Model file for the job. Use its own axes, mm. A direction names the side the tool comes from. Round coordinates to 2 decimals unless told otherwise and drop trailing zeros. Loops run counter-clockwise (first coordinate to the right, second up) from the corner with the lowest first, then second, coordinate; pieces in that order, holes last.
Autodesk Inventor part; units mm, degrees
ref_plane "YZ Plane" through (0, 0, 0) normal (1, 0, 0) x (0, 1, 0)
ref_plane "XZ Plane" through (0, 0, 0) normal (0, 1, 0) x (-1, 0, 0)
ref_plane "XY Plane" through (0, 0, 0) normal (0, 0, 1) x (1, 0, 0)
sketch "Sketch1" plane through (0, 0, 0) normal (0, 1, 0) x (-1, 0, 0)
  circle A0 centre (0, 0) radius 14.986
  dimension "d0" = 29.972
extrude "Extrusion1" add sketch "Sketch1" along normal mid plane 99.06
sketch "Sketch2" plane through (0, 0, 0) normal (1, 0, 0) x (0, 1, 0)
  line L0 (-49.53, 14.986) -> (-49.53, -14.986)
  line L1 (49.53, -14.986) -> (49.53, 14.986)
  line L2 (0, 14.986) -> (0, -71.9195) construction
  line L3 (49.53, 14.986) -> (49.53, -46.736)
  line L4 (49.53, -46.736) -> (111.252, -46.736)
  line L5 (111.252, -46.736) -> (49.53, 14.986)
  line L6 (-49.53, -14.986) -> (-49.53, 14.986)
  line L7 (-49.53, 14.986) -> (-49.53, -46.736)
  line L8 (-49.53, -46.736) -> (-111.252, -46.736)
  line L9 (-111.252, -46.736) -> (-49.53, 14.986)
  point P0 (0, 0)
  dimension "d3" = 61.722
  dimension "d4" = 61.722
extrude "Extrusion2" add sketch "Sketch2" along normal mid plane 25.4
sketch "Sketch3" plane through (12.7, 111.252, -46.736) normal (0, 0, -1) x (-1, 0, 0)
  line L0 (12.7, -111.252) -> (12.7, -6.477) construction
  circle A0 centre (12.7, -6.477) radius 58.42
  line L1 (12.7, -111.252) -> (-79.2707, -111.252) construction
  circle A1 centre (12.7, -216.027) radius 58.42
  dimension "d7" = 104.775
  dimension "d8" = 116.84
extrude "Extrusion3" add sketch "Sketch3" along normal blind 3.81
equation "\"d4\" = d3"
properties part number "SuctionCup"
Q1. Slice it at A-A on x = 45. Give the cut face in (y, z), plus the area to 3 significant figures.
Q2. Probe line 1 (Z direction, x = -23, y = 101); line 2 (Y direction, x = 4, z = -33); line 3 (X direction, y = 53, z = -37). List the from-to ranges inside material, lowest first.
Q3. Tool access for faces 5 (the face through (1.95, -0.69, -14.86)), 6 (the face through (-10, 49.53, 13)), 7 (the face through (10, -49.53, 13)), 8 (the face through (-0.178, 80.823, -16.307)): list every direction of +Z, -Z, +X, -X, +Y, -Y with a clear straight run to the whole face (end or side of a thin tool).
Q4. Slice it at B-B on z = -32.5. Give the cut face in (x, y), plus the area to 3 significant figures.
Q5. Flat gauge pins, fed straight in: P1, Ø6, axis at y = -78.5, z = -27.5, coming from the -X side; P2, Ø3.5, axis at x = 6, z = 11.5, coming from the +Y side; P3, Ø2, axis at x = -8.5, z = 12, coming from the -Y side. Where does each tip first touch, or does it go through?
Q6. Slice it at C-C on y = 99. Give the cut face in (x, z).
Q7. Slice it at D-D on x = -7.5. Give the cut face in (y, z), plus the area to 3 significant figures.
Q8. Pull direction Z, two halves, no side cores. Call faces 1 (the face through (-0.178, -80.823, -16.307)), 2 (the face through (-10, -49.53, 13)), 3 (the face through (0, -49.53, -31)), 4 (the face through (1, -104, -50.546)): pulls with the +Z half, pulls with the -Z half, needs draft (parallel to the pull), parting line crosses it, or undercut.
Reply:
1. outline: (-142.03, -50.55) - (-67.52, -50.55) - (-67.52, -46.74) - (-142.03, -46.74) - close; (67.52, -50.55) - (142.03, -50.55) - (142.03, -46.74) - (67.52, -46.74) - close
1. area: 568 mm2
2. line 1: z = -50.55 to -46.74
2. line 2: y = -97.52 to -49.53, 49.53 to 97.52
2. line 3: x = -12.7 to 12.7
3. face 5: none
3. face 6: +Z, -X
3. face 7: +Z, +X
3. face 8: +Z, +X, -X, +Y
4. outline: (-12.7, -97.02) - (12.7, -97.02) - (12.7, -49.53) - (-12.7, -49.53) - close; (-12.7, 49.53) - (12.7, 49.53) - (12.7, 97.02) - (-12.7, 97.02) - close
4. area: 2,410 mm2
5. P1: stops at x = -12.7
5. P2: stops at y = 54.77
5. P3: stops at y = -53.52
6. outline: (-58.13, -50.55) - (58.13, -50.55) - (58.13, -46.74) - (12.7, -46.74) - (12.7, -34.48) - (-12.7, -34.48) - (-12.7, -46.74) - (-58.13, -46.74) - close
7. outline: (-162.71, -50.55) - (-46.84, -50.55) - (-46.84, -46.74) - (-49.53, -46.74) - (-49.53, -12.97) - (49.53, -12.97) - (49.53, -46.74) - (46.84, -46.74) - (46.84, -50.55) - (162.71, -50.55) - (162.71, -46.74) - (111.25, -46.74) - (49.53, 14.99) - (49.53, 12.97) - (-49.53, 12.97) - (-49.53, 14.99) - (-111.25, -46.74) - (-162.71, -46.74) - close
7. area: 7,260 mm2
8. face 1: pulls with the +Z half
8. face 2: needs draft
8. face 3: undercut
8. face 4: pulls with the -Z half
